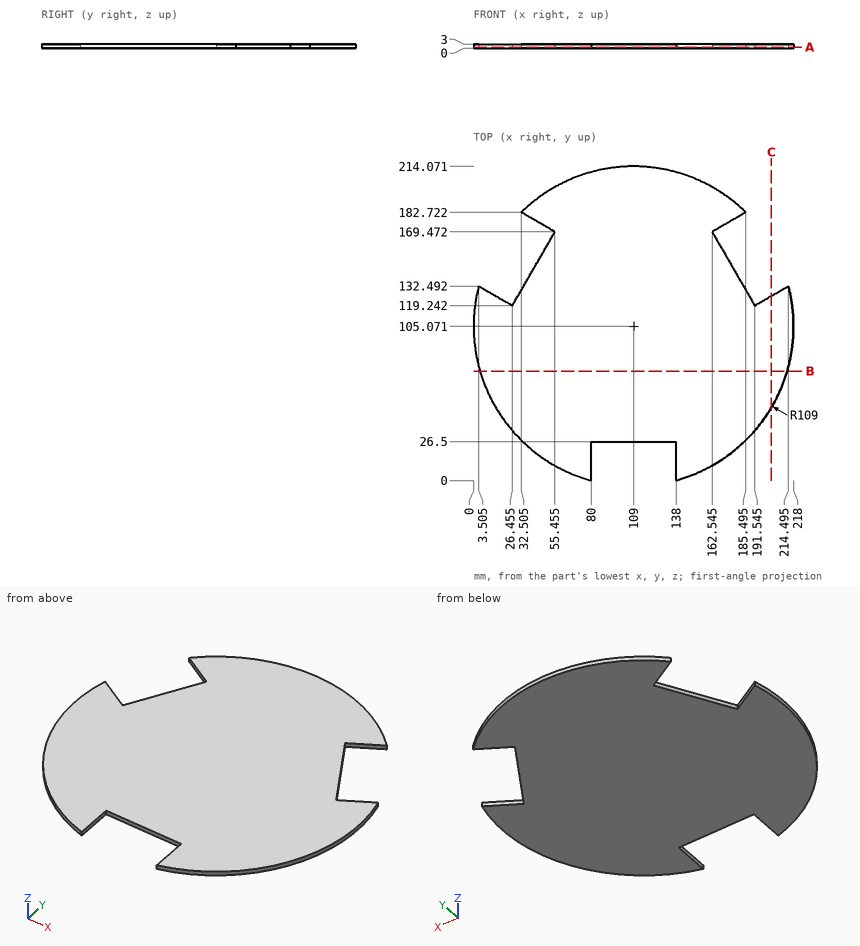
Can you work these out from the drawing? Everything is in mm from the part's minimum corner. Coordinates: 2 decimals unless noted, no trailing zeros. Write each loop counter-clockwise with the first axis right and the second up, starting at its lowest first coordinate (ties: lowest second). Pieces come first, ordered by that corner, then holes. Notation, with made-up numbers: (-29.5, -5) - (16.5, -5) arc R14 ccw to (16.5, 0) - close; hole circle Ø6 at (-21.5, -14). An arc over 180 degrees is marked (long way). One line per item, written item: value.
1) I need wall thicknesses on line 1 along X through (y, z) = (14, 1.5) (1 decimal); line 2 along Y through (x, z) = (37.5, 2.2) (1 decimal); line 3 along X through (y, z) = (168.5, 0.9) (1 decimal). Which ranges of each line are inside material? Lowest first, please.
Model answer:
line 1: x = 49.1 to 80, 138 to 168.9
line 2: y = 22.8 to 138.4, 179.8 to 187.3
line 3: x = 54.9 to 163.1
2) I'm going to push flat-ended pins straight in: P1, Ø0.9, axis at y = 7, z = 1.5, coming from the -X side (1 decimal); P2, Ø1.5, axis at x = 106, z = 2, coming from the -Y side; P3, Ø1.5, axis at x = 115.5, y = 69, coming from the -Z side; P4, Ø1, axis at y = 158.5, z = 2, coming from the -X side. Where does each tip first touch, or does it pass through?
Model answer:
P1: stops at x = 60.5
P2: stops at y = 26.5
P3: stops at z = 0
P4: stops at x = 48.83
3) Suppose I cut it at B-B on y = 74.5. Write out the boundary of the cut face in (x, z) (1 decimal).
Model answer:
outline: (4.4, 0) - (213.6, 0) - (213.6, 3) - (4.4, 3) - close
4) Suppose I cut it at C-C on x = 203. Write out the boundary of the cut face in (y, z), and give its area (3 significant figures).
Model answer:
outline: (49.89, 0) - (125.86, 0) - (125.86, 3) - (49.89, 3) - close
area: 228 mm²
5) Suppose I cut it at A-A on z = 0.9. Write out the boundary of the cut face in (x, y) (1 decimal).
Model answer:
outline: (3.5, 132.5) arc R109 ccw to (80, 0) - (80, 26.5) - (138, 26.5) - (138, 0) arc R109 ccw to (214.5, 132.5) - (191.5, 119.2) - (162.5, 169.5) - (185.5, 182.7) arc R109 ccw to (32.5, 182.7) - (55.5, 169.5) - (26.5, 119.2) - close
